```python
from build123d import *
from build123d.topology import SkipClean

# Parameters (mm, degrees)
SKETCH1_W                                            = 177.8
SKETCH1_H                                            = 177.8
BOSS_EXTRUDE1_DEPTH                                  = 12.7
SKETCH2_R                                            = 76.596875
CUT_EXTRUDE1_DEPTH                                   = 19.84375
SKETCH3_R                                            = 6.35
CUT_EXTRUDE2_DEPTH                                   = 19.84375
SKETCH5_W                                            = 12.7
SKETCH5_H                                            = 6.35
CUT_EXTRUDE3_DEPTH                                   = 19.84375
FILLET1_R                                            = 6.35
FILLET2_R                                            = 0.635
FILLET3_R                                            = 0.508
CHAMFER2_SIZE                                        = 1.27
FILLET5_R                                            = 0.762
CBORE_FOR_1_4_BINDING_HEAD_MACHINE_SCREW_D           = 6.7564
CBORE_FOR_1_4_BINDING_HEAD_MACHINE_SCREW_CBORE_D     = 14.2875
CBORE_FOR_1_4_BINDING_HEAD_MACHINE_SCREW_CBORE_DEPTH = 4.191


with BuildPart() as part:
    # Sketch1 → Boss-Extrude1 (new, symmetric)
    with BuildSketch(Plane.XY):
        Rectangle(SKETCH1_W, SKETCH1_H)
    extrude(amount=BOSS_EXTRUDE1_DEPTH, both=True)

    # Sketch2 → Cut-Extrude1 (cut)
    with BuildSketch(Plane.XY.offset(12.7)):
        Circle(SKETCH2_R)
    extrude(amount=-CUT_EXTRUDE1_DEPTH, mode=Mode.SUBTRACT)

    # Sketch3 → Cut-Extrude2 (cut)
    with BuildSketch(Plane.XY.offset(-7.14375)):
        Circle(SKETCH3_R)
    extrude(amount=-CUT_EXTRUDE2_DEPTH, mode=Mode.SUBTRACT)

    # Sketch5 → Cut-Extrude3 (cut)
    with SkipClean():  # the faces are left unmerged after this step: merging them gives an invalid solid
        with BuildSketch(Plane.XY.offset(-7.14375)):
            with BuildLine():
                Line((-73.421875, 21.824516747), (-73.421875, -21.824516747))
                ThreePointArc((-73.421875, -21.824516747), (-76.596875, 0), (-73.421875, 21.824516747))
            make_face()
            with Locations((0, 73.533)):
                Rectangle(SKETCH5_W, SKETCH5_H)
            with BuildLine():
                Line((63.896875, 30.068721747), (63.896875, -30.068721747))
                Line((63.896875, -30.068721747), (70.448230867, -30.068721747))
                ThreePointArc((70.448230867, -30.068721747), (76.596875, 0), (70.448230867, 30.068721747))
                Line((70.448230867, 30.068721747), (63.896875, 30.068721747))
            make_face()
        extrude(amount=-CUT_EXTRUDE3_DEPTH, mode=Mode.SUBTRACT)

    # Fillet1
    fillet1_edges = [part.edges().sort_by_distance(p)[0] for p in [
        (88.9, 88.9, 0),
        (88.9, -88.9, 0),
        (-88.9, -88.9, 0),
        (-88.9, 88.9, 0),
    ]]
    fillet(fillet1_edges, radius=FILLET1_R)

    # Fillet2
    # the kernel refuses this fillet: 0.635 mm, written as the material it adds along each edge
    with BuildSketch(Plane(origin=(-6.35, 76.708, -7.14375), x_dir=(0, -1, 0), z_dir=(0, 0, -1))) as fillet2_piece_1:
        with BuildLine():
            CenterArc((FILLET2_R, -FILLET2_R), FILLET2_R, 90, 90)
            Line((0, -FILLET2_R), (0, 0))
            Line((0, 0), (FILLET2_R, 0))
        make_face()
    extrude(amount=5.55625)
    with BuildSketch(Plane(origin=(-6.35, 70.358, -7.14375), x_dir=(0, 1, 0), z_dir=(0, 0, -1)), Plane(origin=(6.35, 76.708, -7.14375), x_dir=(0, -1, 0), z_dir=(0, 0, -1)), Plane(origin=(6.35, 70.358, -7.14375), x_dir=(-1, 0, 0), z_dir=(0, 0, -1))) as fillet2_piece_2:
        with BuildLine():
            CenterArc((FILLET2_R, FILLET2_R), FILLET2_R, 180, 90)
            Line((0, FILLET2_R), (0, 0))
            Line((0, 0), (FILLET2_R, 0))
        make_face()
    extrude(amount=5.55625)

    # Fillet3
    # the kernel refuses this fillet: 0.508 mm, written as the material it adds along each edge
    with BuildSketch(Plane(origin=(-73.421875, -21.824516747, -7.14375), x_dir=(0, 1, 0), z_dir=(0, 0, -1))) as fillet3_piece_1:
        with BuildLine():
            CenterArc((3.827559192, -0.508), FILLET3_R, 90, 166.318438428)
            ThreePointArc((3.707404249, -1.001585646), (1.847424112, -0.524031105), (0, 0))
            Line((0, 0), (3.827559192, 0))
        make_face()
    extrude(amount=5.55625)
    with BuildSketch(Plane(origin=(-73.421875, 21.824516747, -7.14375), x_dir=(0, -1, 0), z_dir=(0, 0, -1))) as fillet3_piece_2:
        with BuildLine():
            CenterArc((3.827559192, 0.508), FILLET3_R, 103.681561572, 166.318438428)
            ThreePointArc((3.707404249, 1.001585646), (1.847424112, 0.524031105), (0, 0))
            Line((0, 0), (3.827559192, 0))
        make_face()
    extrude(amount=5.55625)

    # Chamfer2
    chamfer2_edges = [part.edges().sort_by_distance(p)[0] for p in [
        (-6.35, 0, -12.7),
        (-6.35, 0, -7.14375),
    ]]
    chamfer(chamfer2_edges, length=CHAMFER2_SIZE)

    # Fillet5
    # the kernel refuses this fillet: 0.762 mm, written as the material it adds along each edge
    with BuildSketch(Plane(origin=(70.448230867, -30.068721747, -7.14375), x_dir=(-1, 0, 0), z_dir=(0, 0, -1))) as fillet5_piece_1:
        with BuildLine():
            CenterArc((0.505080189, 0.762), FILLET5_R, 202.734061429, 67.265938571)
            ThreePointArc((-0.197718896, 0.467521741), (-0.099246736, 0.233597083), (0, 0))
            Line((0, 0), (0.505080189, 0))
        make_face()
    extrude(amount=5.55625)
    with BuildSketch(Plane(origin=(63.896875, -30.068721747, -7.14375), x_dir=(1, 0, 0), z_dir=(0, 0, -1)), Plane(origin=(63.896875, 30.068721747, -7.14375), x_dir=(0, -1, 0), z_dir=(0, 0, -1))) as fillet5_piece_2:
        with BuildLine():
            CenterArc((FILLET5_R, -FILLET5_R), FILLET5_R, 90, 90)
            Line((0, -FILLET5_R), (0, 0))
            Line((0, 0), (FILLET5_R, 0))
        make_face()
    extrude(amount=5.55625)
    with BuildSketch(Plane(origin=(70.448230867, 30.068721747, -7.14375), x_dir=(-1, 0, 0), z_dir=(0, 0, -1))) as fillet5_piece_3:
        with BuildLine():
            CenterArc((0.505080189, -0.762), FILLET5_R, 90, 67.265938571)
            ThreePointArc((-0.197718896, -0.467521741), (-0.099246736, -0.233597083), (0, 0))
            Line((0, 0), (0.505080189, 0))
        make_face()
    extrude(amount=5.55625)

    # CBORE for 1/4 Binding Head Machine Screw1 (through all)
    with Locations(Plane(origin=(0, 0, -12.7), x_dir=(-1, 0, 0), z_dir=(0, 0, -1))):
        with Locations((-82.55, 82.55), (82.55, 82.55), (82.55, -82.55), (-82.55, -82.55)):
            CounterBoreHole(CBORE_FOR_1_4_BINDING_HEAD_MACHINE_SCREW_D / 2, CBORE_FOR_1_4_BINDING_HEAD_MACHINE_SCREW_CBORE_D / 2, CBORE_FOR_1_4_BINDING_HEAD_MACHINE_SCREW_CBORE_DEPTH)


solid = part.part
```
The listing builds one solid part. Answer for the finished solid, in the listing's coordinates (mm). A direction names the side the tool comes from. Coordinates: 2 decimals unless noted, no trailing zeros. Write each loop counter-clockwise with the first axis right and the second up, starting at its lowest first coordinate (ties: lowest second). Pieces come first, ordered by that corner, then holes.
Q1. Find the intervals of material crossed by line 1 along Y through (x, z) = (-82.55, -2.5); line 2 along X through (y, z) = (74.5, -8); line 3 along Z through (x, y) = (62.5, -0.5), in increasing order.
Returned:
line 1: y = -88.9 to -85.93, -79.17 to 79.17, 85.93 to 88.9
line 2: x = -88.9 to -6.35, 6.35 to 88.9
line 3: z = -12.7 to -7.14
Q2. Given P1, Ø11, axis at x = -82.55, y = -82.55, coming from the -Z side; P2, Ø5, axis at x = 36.5, y = 52, coming from the +Z side, each flat-ended and moving along its own axis, determine where each tip first touches the part or whether it passes through.
Returned:
P1: stops at z = -8.51
P2: stops at z = -7.14
Q3. Section C-C, the plane y = 46 is taken. Write down the section's boundary in (x, z).
Returned:
outline: (-88.9, -12.7) - (88.9, -12.7) - (88.9, 12.7) - (61.25, 12.7) - (61.25, -7.14) - (-61.25, -7.14) - (-61.25, 12.7) - (-88.9, 12.7) - close
Q4. Section B-B, the plane z = 5 is taken. Write down the section's boundary in (x, y), then the cut area to 3 significant figures.
Returned:
outline: (-88.9, -82.55) arc R6.35 ccw to (-82.55, -88.9) - (82.55, -88.9) arc R6.35 ccw to (88.9, -82.55) - (88.9, 82.55) arc R6.35 ccw to (82.55, 88.9) - (-82.55, 88.9) arc R6.35 ccw to (-88.9, 82.55) - close; hole circle Ø6.76 at (-82.55, -82.55); hole circle Ø6.76 at (-82.55, 82.55); hole circle Ø153.19 at (0, 0); hole circle Ø6.76 at (82.55, -82.55); hole circle Ø6.76 at (82.55, 82.55)
area: 13,000 mm2
Q5. The mould has two halves that part along Y. Classify faces 1 (the cylindrical face through (-87.09, -86.99, 2.24)), 2 (the flat face through (88.9, -1, 0)), 3 (the flat face through (-79, -82, -8.509)): released by +Y, released by -Y, zero draft, split by the parting line, or undercut.
Returned:
face 1: released by -Y
face 2: zero draft
face 3: undercut
Q6. Which of the six approach directions +Z, -Z, +X, -X, +Y, -Y give full straight-line access (tool end or side, diameter ignored) to faces 4 (the flat face through (67, 30.069, -10)), 5 (the flat face through (78, 1, 12.7)), 6 (the cylindrical face through (-77.6, -77.4, -10.6))?
Returned:
face 4: +Z, -Z
face 5: +Z, +X, -X, +Y, -Y
face 6: -Z
Q7. Section D-D, the plane x = -30 is taken. Write down the section's boundary in (y, z), then the cut area to 3 significant figures.
Returned:
outline: (-88.9, -12.7) - (88.9, -12.7) - (88.9, 12.7) - (70.48, 12.7) - (70.48, -7.14) - (-70.48, -7.14) - (-70.48, 12.7) - (-88.9, 12.7) - close
area: 1,720 mm2
Q8. Section A-A, the plane x = 0 is taken. Write down the section's boundary in (y, z), then the cut area to 3 significant figures.
Returned:
outline: (-88.9, -12.7) - (-7.62, -12.7) - (-6.35, -11.43) - (-6.35, -8.41) - (-7.62, -7.14) - (-76.6, -7.14) - (-76.6, 12.7) - (-88.9, 12.7) - close; (6.35, -11.43) - (7.62, -12.7) - (70.36, -12.7) - (70.36, -7.14) - (7.62, -7.14) - (6.35, -8.41) - close; (76.6, -7.14) - (76.71, -7.14) - (76.71, -12.7) - (88.9, -12.7) - (88.9, 12.7) - (76.6, 12.7) - close
area: 1,370 mm2
